The listing builds one solid part. Answer for the finished solid, in the listing's coordinates (mm). Face numbers are marked on the shaded views. A direction names the side the tool comes from. Give positions to 0.01 mm unless a question says otherwise; leave off trailing zeros. Write each loop counter-clockwise with the first axis right and the second up, starting at its lowest first coordinate (ties: lowest second). Pieces come first, ordered by that corner, then holes.
```python
from build123d import *

# Parameters (mm, degrees)
SKETCH1_W               = 38.1
SKETCH1_H               = 50.673
BOSS_EXTRUDE1_DEPTH     = 3.175
CUT_EXTRUDE1_REACH      = 34.329
SKETCH2_W               = 12.7
SKETCH2_H               = 6.35
MIRROR2_COPY_1_REACH    = 34.329
MIRROR2_COPY_1_SKETCH_W = 12.7
MIRROR2_COPY_1_SKETCH_H = 6.35
F_1_4_CLEARANCE_HOLE1_D = 6.7564


with BuildPart() as part:
    # Sketch1 → Boss-Extrude1 (new, symmetric)
    with BuildSketch(Plane(origin=(0, 0, 0), x_dir=(0, 0, -1), z_dir=(1, 0, 0))):
        Rectangle(SKETCH1_W, SKETCH1_H)
    extrude(amount=BOSS_EXTRUDE1_DEPTH, both=True)

    # Sketch2 → Cut-Extrude1 (cut, up to next)
    with BuildSketch(Plane(origin=(3.175, 0, 0), x_dir=(0, 0, -1), z_dir=(1, 0, 0)), mode=Mode.PRIVATE) as cut_extrude1_sk1:
        with Locations((-12.7, 22.1615)):
            Rectangle(SKETCH2_W, SKETCH2_H)
    cut_extrude1_tool1 = extrude(cut_extrude1_sk1.sketch, amount=-CUT_EXTRUDE1_REACH, mode=Mode.PRIVATE) & part.part
    cut_extrude1 = cut_extrude1_tool1.solids().sort_by_distance((3.175, 22.1615, 12.7))[0]
    add(cut_extrude1, mode=Mode.SUBTRACT)

    # Mirror1: Cut-Extrude1 across plane
    add(cut_extrude1.mirror(Plane.XY), mode=Mode.SUBTRACT)

    # Sketch3 → #6 Clearance Hole1 (revolve, cut)
    with BuildSketch(Plane(origin=(3.175, 22.1615, 0), x_dir=(0, 0, -1), z_dir=(0, 1, 0))):
        Polygon((0, 0), (0, 10.030824014), (1.89865, 8.89), (1.89865, 0), align=None)
    f_6_clearance_hole1 = revolve(axis=Axis((9.525, 22.1615, 0), (-1, 0, 0)), mode=Mode.SUBTRACT)

    # Mirror2: Cut-Extrude1, #6 Clearance Hole1 across plane
    add(cut_extrude1.mirror(Plane.ZX), mode=Mode.SUBTRACT)
    add(f_6_clearance_hole1.mirror(Plane.ZX), mode=Mode.SUBTRACT)

    # Mirror2 copy 1 sketch → Mirror2 copy 1 (cut, up to next)
    with BuildSketch(Plane(origin=(3.175, 0, 0), x_dir=(0, 0, 1), z_dir=(1, 0, 0)), mode=Mode.PRIVATE) as mirror2_copy_1_sk1:
        with Locations((-12.7, 22.1615)):
            Rectangle(MIRROR2_COPY_1_SKETCH_W, MIRROR2_COPY_1_SKETCH_H)
    mirror2_copy_1_tool1 = extrude(mirror2_copy_1_sk1.sketch, amount=-MIRROR2_COPY_1_REACH, mode=Mode.PRIVATE) & part.part
    add(mirror2_copy_1_tool1.solids().sort_by_distance((3.175, -22.1615, -12.7))[0], mode=Mode.SUBTRACT)

    # 1/4 Clearance Hole1 (through all)
    with Locations(Plane(origin=(3.175, 0, 0), x_dir=(0, 0, -1), z_dir=(1, 0, 0))):
        with Locations((0, 0)):
            Hole(F_1_4_CLEARANCE_HOLE1_D / 2)


solid = part.part
```
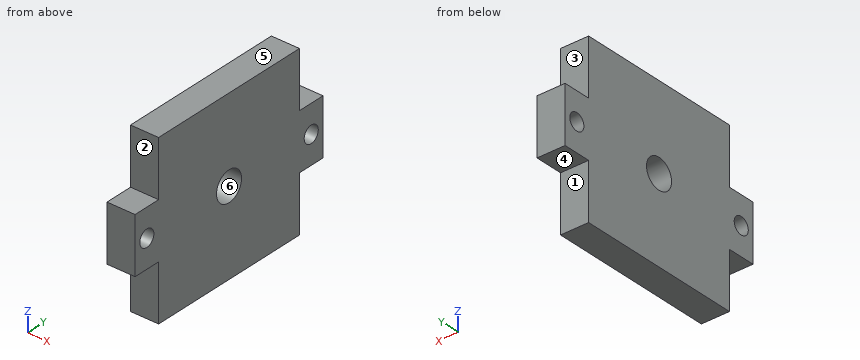
Item 1: Each of these flat-tipped pins is pushed along its axis until it touches: P1, Ø1, axis at x = 2, y = -20, coming from the +Z side; P2, Ø1.5, axis at x = -0.5, z = -9, coming from the +Y side; P3, Ø1.9, axis at x = -0.5, y = 21, coming from the -Z side. Where does it stop, or does it pass through?
Conclusion:
P1: stops at z = 6.35
P2: stops at y = 18.99
P3: stops at z = -6.35
Item 2: A cutting plane is placed at C-C, the plane x = 1. Give the vertices of the cut face in (y, z), plus the area to 3 significant figures.
Conclusion:
outline: (-25.34, -6.35) - (-18.99, -6.35) - (-18.99, -19.05) - (18.99, -19.05) - (18.99, -6.35) - (25.34, -6.35) - (25.34, 6.35) - (18.99, 6.35) - (18.99, 19.05) - (-18.99, 19.05) - (-18.99, 6.35) - (-25.34, 6.35) - close; hole circle Ø3.8 at (-22.16, 0); hole circle Ø6.76 at (0, 0); hole circle Ø3.8 at (22.16, 0)
area: 1,550 mm2
Item 3: Consider probe 1 along Y at (x, z) = (-1, 0); probe 2 along Y at (x, z) = (0, 17); probe 3 along Z at (x, y) = (-1, 3). Determine where each line is inside the solid, lowest interval first.
Conclusion:
probe 1: y = -25.34 to -24.06, -20.26 to -3.38, 3.38 to 20.26, 24.06 to 25.34
probe 2: y = -18.99 to 18.99
probe 3: z = -19.05 to -1.55, 1.55 to 19.05
Item 4: A cutting plane is placed at D-D, the plane z = 12. Give the vertices of the cut face in (x, y) (1 decimal).
Conclusion:
outline: (-3.2, -19) - (3.2, -19) - (3.2, 19) - (-3.2, 19) - close
Item 5: A cutting plane is placed at A-A, the plane y = 0. Give the vertices of the cut face in (x, z) (3 decimals).
Conclusion:
outline: (-3.175, -19.05) - (3.175, -19.05) - (3.175, -3.378) - (-3.175, -3.378) - close; (-3.175, 3.378) - (3.175, 3.378) - (3.175, 19.05) - (-3.175, 19.05) - close
Item 6: Which of the six approach directions +Z, -Z, +X, -X, +Y, -Y give full straight-line access (tool end or side, diameter ignored) to the marked faces 1, 2 and 3?
Conclusion:
face 1: -Z, +X, -X, +Y
face 2: +Z, +X, -X, -Y
face 3: +Z, +X, -X, +Y
Item 7: Determine the mould class of the marked faces 4, 5 and 6 for opening direction Z: pulls with the +Z half, pulls with the -Z half, needs draft (parallel to the pull), parting line crosses it, or undercut.
Conclusion:
face 4: pulls with the -Z half
face 5: pulls with the +Z half
face 6: undercut
Item 8: A cutting plane is placed at B-B, the plane z = 0. Give the vertices of the cut face in (x, y) (1 decimal).
Conclusion:
outline: (-3.2, -25.3) - (3.2, -25.3) - (3.2, -24.1) - (-3.2, -24.1) - close; (-3.2, -20.3) - (3.2, -20.3) - (3.2, -3.4) - (-3.2, -3.4) - close; (-3.2, 3.4) - (3.2, 3.4) - (3.2, 20.3) - (-3.2, 20.3) - close; (-3.2, 24.1) - (3.2, 24.1) - (3.2, 25.3) - (-3.2, 25.3) - close
